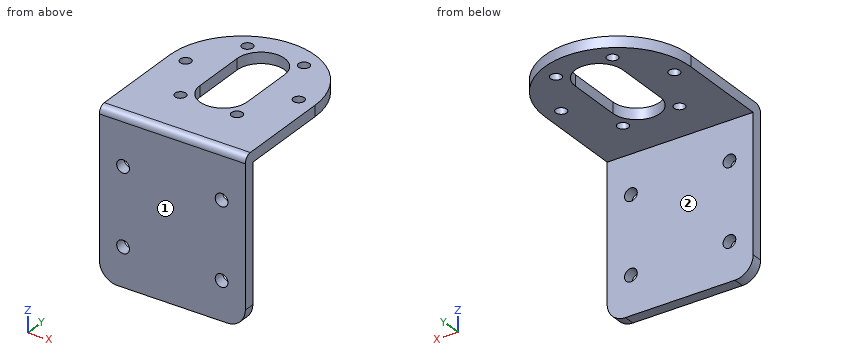
```python
from build123d import *

# Parameters (mm, degrees)
CROQUIS1_R              = 1.5
SALIENTE_EXTRUIR1_DEPTH = 1.5
CORTAR_EXTRUIR3_DEPTH   = 3
CROQUIS3_W              = 40
CROQUIS3_H              = 3
SALIENTE_EXTRUIR2_DEPTH = 42.2
CROQUIS4_R              = 1.75
CORTAR_EXTRUIR5_DEPTH   = 42.2
REDONDEO1_R             = 2
REDONDEO2_R             = 5


with BuildPart() as part:
    # Croquis1 → Saliente-Extruir1 (new, symmetric)
    with BuildSketch(Plane.XY):
        with BuildLine():
            Line((-20, -24), (20, -24))
            Line((20, -24), (20, 4))
            ThreePointArc((20, 4), (0, 24), (-20, 4))
            Line((-20, 4), (-20, -24))
        make_face()
        with Locations((-15.5, 4)):
            Circle(CROQUIS1_R, mode=Mode.SUBTRACT)
        with Locations((-7.75, 17.423393759)):
            Circle(CROQUIS1_R, mode=Mode.SUBTRACT)
        with Locations((7.75, 17.423393759)):
            Circle(CROQUIS1_R, mode=Mode.SUBTRACT)
        with Locations((15.5, 4)):
            Circle(CROQUIS1_R, mode=Mode.SUBTRACT)
        with Locations((7.75, -9.423393759)):
            Circle(CROQUIS1_R, mode=Mode.SUBTRACT)
        with Locations((-7.75, -9.423393759)):
            Circle(CROQUIS1_R, mode=Mode.SUBTRACT)
    extrude(amount=SALIENTE_EXTRUIR1_DEPTH, both=True)

    # Croquis2 → Cortar-Extruir3 (cut)
    with BuildSketch(Plane.XY.offset(1.5)):
        with BuildLine():
            Line((6.5, 11.5), (6.5, -3.5))
            ThreePointArc((6.5, -3.5), (0, -10), (-6.5, -3.5))
            Line((-6.5, -3.5), (-6.5, 11.5))
            ThreePointArc((-6.5, 11.5), (0, 18), (6.5, 11.5))
        make_face()
    extrude(amount=-CORTAR_EXTRUIR3_DEPTH, mode=Mode.SUBTRACT)

    # Croquis3 → Saliente-Extruir2 (add)
    with BuildSketch(Plane(origin=(0, 0, -1.5), x_dir=(-1, 0, 0), z_dir=(0, 0, -1))):
        with Locations((0, -22.5)):
            Rectangle(CROQUIS3_W, CROQUIS3_H)
    extrude(amount=SALIENTE_EXTRUIR2_DEPTH)

    # Croquis4 → Cortar-Extruir5 (cut)
    with BuildSketch(Plane(origin=(0, -21, 0), x_dir=(1, 0, 0), z_dir=(0, 1, 0))):
        with Locations(Location((-13.5, 33.1, 0), (0, 0, 270))):
            Circle(CROQUIS4_R)
        with Locations(Location((13.5, 33.1, 0), (0, 0, 270))):
            Circle(CROQUIS4_R)
        with Locations(Location((13.5, 12.1, 0), (0, 0, 270))):
            Circle(CROQUIS4_R)
        with Locations(Location((-13.5, 12.1, 0), (0, 0, 270))):
            Circle(CROQUIS4_R)
    extrude(amount=-CORTAR_EXTRUIR5_DEPTH, mode=Mode.SUBTRACT)

    # Redondeo1
    redondeo1_edges = [part.edges().sort_by_distance(p)[0] for p in [
        (0, -24, 1.5),
    ]]
    fillet(redondeo1_edges, radius=REDONDEO1_R)

    # Redondeo2
    redondeo2_edges = [part.edges().sort_by_distance(p)[0] for p in [
        (20, -22.5, -43.7),
        (-20, -22.5, -43.7),
    ]]
    fillet(redondeo2_edges, radius=REDONDEO2_R)


solid = part.part
```
Here's how the part is built. I have some questions about the finished solid (model axes, mm). Face numbers are marked on the shaded views. A direction names the side the tool comes from. Give positions to 0.01 mm unless a question says otherwise; leave off trailing zeros. Loops run counter-clockwise (first coordinate to the right, second up) from the corner with the lowest first, then second, coordinate; pieces in that order, holes last. Notation, with made-up numbers: (28.25, 4) -> (84.25, 4) arc R13 ccw to (84.25, 27) -> close; hole circle Ø3 at (85, 7). An arc over 180 degrees is marked (long way). Use one line per item in the form item = value. Start each with the question number.
1) Imagine slicing it at D-D (z = -7). Please give me the cut outline in (x, y).
2) Please list where these lines run through material, in increasing order: line 1 along X through (y, z) = (-23, -33); line 2 along Y through (x, z) = (7.75, -0.6); line 3 along Z through (x, y) = (4, 18).
3) Imagine slicing it at B-B (y = 1). Please give me the cut outline in (x, z), then the cut area to 3 significant figures.
4) Imagine slicing it at C-C (x = -7.75). Please give me the cut outline in (y, z).
5) Imagine slicing it at A-A (z = -12.1). Please give me the cut outline in (x, y), then the cut area to 3 significant figures.
6) Which directions (+Z, -Z, +X, -X, +Y, -Y) give clear straight access to the entire face, cutting with the end or side of a thin tool? Please do the marked faces 1 and 2.
7) For P1, Ø0.9, axis at y = 7.5, z = 0.5, coming from the +X side; P2, Ø10, axis at x = -4, z = -12, coming from the +Y side; P3, Ø5, axis at x = 15.5, y = 4, coming from the +Z side; P4, Ø12, axis at x = -14.5, y = -0.5, coming from the -Z side, each with a flat end and sliding along its axis, tell me the tip position at first contact or that it passes through.
Check values:
q1.outline = (-20, -24) -> (20, -24) -> (20, -21) -> (-20, -21) -> close
q2.line_1 = -20 to -15.25, -11.75 to 11.75, 15.25 to 20
q2.line_2 = -24 to -10.92, -7.92 to 15.92, 18.92 to 22.44
q2.line_3 = -1.5 to 1.5
q3.outline = (-20, -1.5) -> (-6.5, -1.5) -> (-6.5, 1.5) -> (-20, 1.5) -> close; (6.5, -1.5) -> (20, -1.5) -> (20, 1.5) -> (6.5, 1.5) -> close
q3.area = 81.0 mm^2
q4.outline = (-24, -43.7) -> (-21, -43.7) -> (-21, -1.5) -> (-10.92, -1.5) -> (-10.92, 1.5) -> (-22, 1.5) arc R2 ccw to (-24, -0.5) -> close; (-7.92, -1.5) -> (15.92, -1.5) -> (15.92, 1.5) -> (-7.92, 1.5) -> close; (18.92, -1.5) -> (22.44, -1.5) -> (22.44, 1.5) -> (18.92, 1.5) -> close
q5.outline = (-20, -24) -> (-15.25, -24) -> (-15.25, -21) -> (-20, -21) -> close; (-11.75, -24) -> (11.75, -24) -> (11.75, -21) -> (-11.75, -21) -> close; (15.25, -24) -> (20, -24) -> (20, -21) -> (15.25, -21) -> close
q5.area = 99.0 mm^2
q6.face_1 = +Z, -Z, +X, -X, -Y
q6.face_2 = -Z, +X, -X, +Y
q7.P1 = 19.77
q7.P2 = -21
q7.P3 = 1.5
q7.P4 = -1.5
